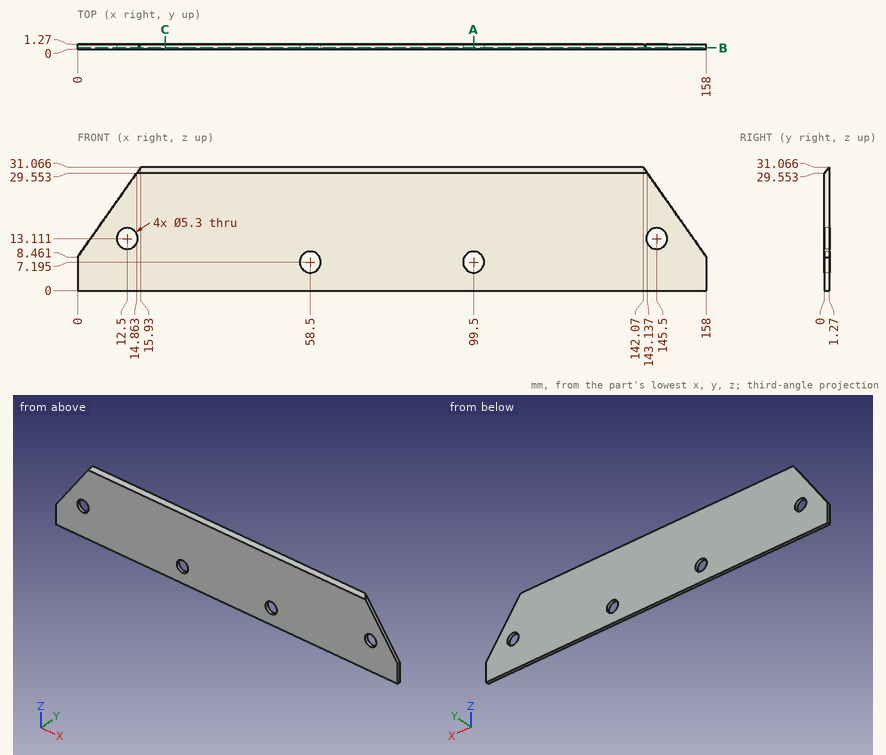
Design review of the part shown in the three views and the two pictorial views. Dimensions are in mm from the part's minimum x, y and z. Round coordinates to 2 decimals unless told otherwise and drop trailing zeros. Loops run counter-clockwise (first coordinate to the right, second up) from the corner with the lowest first, then second, coordinate; pieces in that order, holes last. Notation, with made-up numbers: (-19.75, 24) -> (-15.75, 24) arc R25 cw to (-15.75, 43) -> close; hole circle Ø8 at (16, -9). An arc over 180 degrees is marked (long way). Use one line per item in the form item = value. Start each with the question number.
Q1. We need section C-C on x = 22. Give the boundary of the cut face in (y, z).
Q2. We need section B-B on y = 0.3. State how many separate pieces and enclosed holes the cut face has, then the cut area to 3 significant figures.
Q3. We need section A-A on x = 99.5. Give the boundary of the cut face in (y, z) (1 decimal).
Q4. For pin 1 Ø3 at (x, z) = (58.5, 7.19) entering from +Y; pin 2 Ø6 at (x, z) = (99.5, 7.19) entering from -Y, all flat-tipped, find the tip position at first contact; note any pin that passes through.
Q5. Wall thickness on line 1 along X through (y, z) = (0.7, 7.5); line 2 along X through (y, z) = (0.8, 5) (1 decimal); line 3 along Z through (x, y) = (12.5, 0.3): over which ranges is each line inside the solid? List them lowest first. Write a range as [from, to].
Calculated:
q1.outline = (0, 0) -> (1.27, 0) -> (1.27, 31.07) -> (0, 29.55) -> close
q2.separate_pieces = 1
q2.enclosed_holes = 4
q2.area = 4,310 mm²
q3.outline = (0, 0) -> (1.3, 0) -> (1.3, 4.5) -> (0, 4.5) -> close; (0, 9.8) -> (1.3, 9.8) -> (1.3, 31.1) -> (0, 29.6) -> close
q4.pin_1 = through
q4.pin_2 = 0
q5.line_1 = [0, 55.87], [61.13, 96.87], [102.13, 158]
q5.line_2 = [0, 57], [60, 98], [101, 158]
q5.line_3 = [0, 10.46], [15.76, 26.2]
